```python
from build123d import *

# Parameters (mm, degrees)
F0_R            = 60
F1_DEPTH        = 20
F3_DEPTH        = 20
F3_COPIES_COUNT = 30


# Not quite as in the source:
# - a pattern or mirror of a feature is missing from the dataset's text; its kind, count and spacing are read off the source's solid


with BuildPart() as f1:
    # F0 (on Front) → F1 (new body)
    with BuildSketch(Plane.XZ):
        Circle(F0_R)
    extrude(amount=F1_DEPTH)

    # F2 (on face) → F3 (join)
    with BuildSketch(Plane.XZ.offset(20)):
        Polygon((0, 77.9763460159), (-6.2717077961, 59.6713137221), (6.2717077961, 59.6713137221), align=None)
    f3 = extrude(amount=-F3_DEPTH)

    # F3_copies: F3 ×30 about axis
    f3_copies_axis = Axis((0, 0, 0), (0, 1, 0))
    for i in range(1, F3_COPIES_COUNT):
        add(f3.rotate(f3_copies_axis, i * 360 / F3_COPIES_COUNT))


solid = f1.part
```
The listing builds one solid part. Answer for the finished solid, in the listing's coordinates (mm). A direction names the side the tool comes from. Give positions to 0.01 mm unless a question says otherwise; leave off trailing zeros. Order: outer loops, then holes, each group sorted by start corner. A loop starts at its lowest first (then second) coordinate and runs counter-clockwise, first axis right, second up. Notation, with made-up numbers: (-18.75, 20) -> (8.25, 20) arc R29 ccw to (8.25, 42) -> close; hole circle Ø4 at (-2.5, 50.25). An arc over 180 degrees is marked (long way). Answer as a JSON object with one key per item and string values. Group by question number.
Item 1: The part is cut by section B-B on x = 34.5. Write down the section's boundary in (y, z), and give its area (3 significant figures).
Item 2: The part is cut by section C-C on z = -19. Write down the section's boundary in (x, y).
Item 3: Flat-ended cylindrical pins translate along their axes: pin 1 (8 mm diameter, centred on y = -10, z = 58, fed in from +X); pin 2 (6 mm diameter, centred on y = -2.5, z = 35, fed in from -X); pin 3 (1 mm diameter, centred on y = -14.5, z = 19, fed in from -X). Find the tip coordinate at first contact, or state that the pin passes through.
Item 4: Determine the mould class of faces 1 (the flat face through (-37.806, -10.14, 57.445)), 2 (the flat face through (-68.251, -10.14, -10.282)), 3 (the flat face through (-1, -20, 1)), 4 (the flat face through (66.533, -10.14, -18.367)) for opening direction X: pulls with the +X half, pulls with the -X half, needs draft (parallel to the pull), parting line crosses it, or undercut.
Item 5: A tool of negligible diameter and unlimited length cuts with its end or side. For faces 5 (the flat face through (3.092, -10.14, -68.952)), 6 (the flat face through (58.168, -10.14, 37.154)), 7 (the flat face through (-68.897, -10.14, 4.132)), 8 (the flat face through (68.897, -10.14, -4.132)), 9 (the flat face through (11.312, -10.14, 68.088)), from which of +Z, -Z, +X, -X, +Y, -Y can it reach the whole face along a straight path? Write none if from no direction.
Item 6: The part is cut by section A-A on z = -47.5. Write down the section's boundary in (x, y).
Item 7: Consider L1, parallel to X at y = -2, z = -54; L2, parallel to Z at x = -57.5, y = -1; L3, parallel to X at y = -18, z = -46. Determine where each line is inside the solid, lowest interval first. Write a range as from..to.
Result set:
{
 "1": {"outline": "(-20, -55.12) -> (0, -55.12) -> (0, 55.12) -> (-20, 55.12) -> close", "area": "2,200 mm²"},
 "2": {"outline": "(-67.38, -20) -> (67.38, -20) -> (67.38, 0) -> (-67.38, 0) -> close"},
 "3": {"pin 1": "x = 45.5", "pin 2": "x = -66.67", "pin 3": "x = -68.04"},
 "4": {"face 1": "undercut", "face 2": "pulls with the -X half", "face 3": "needs draft", "face 4": "pulls with the +X half"},
 "5": {"face 5": "-Z, +Y, -Y", "face 6": "+Y, -Y", "face 7": "-X, +Y, -Y", "face 8": "+X, +Y, -Y", "face 9": "+Z, +Y, -Y"},
 "6": {"outline": "(-55.35, -20) -> (-46.98, -20) -> (-46.98, 0) -> (-55.35, 0) -> close; (-41.04, -20) -> (41.04, -20) -> (41.04, 0) -> (-41.04, 0) -> close; (46.98, -20) -> (55.35, -20) -> (55.35, 0) -> (46.98, 0) -> close"},
 "7": {"L1": "-43.04..-32.9, -30.18..30.18, 32.9..43.04", "L2": "-51.99..-51.37, -37.02..-27.49, -24.36..24.36, 27.49..37.02, 51.37..51.99", "L3": "-54.51..-43.46, -40.58..40.58, 43.46..54.51"}
}
